Part model, mm, in its own coordinate system. Face numbers are marked on the shaded views. A direction names the side the tool comes from. Round coordinates to 2 decimals unless told otherwise and drop trailing zeros. Write each loop counter-clockwise with the first axis right and the second up, starting at its lowest first coordinate (ties: lowest second). Pieces come first, ordered by that corner, then holes. Notation, with made-up numbers: (30.25, 6) -> (48.25, 6) arc R11 ccw to (48.25, 19) -> close; hole circle Ø9 at (52, 54.5). An arc over 180 degrees is marked (long way). Use CSV: the item, a comma, the result in double quotes. Start each with the question number.
(1) Two-plate mould, pull along Z, no slides. Class the marked faces 1, 2 and 3: released by +Z, released by -Z, zero draft, split by the parting line, or undercut.
(2) Saw through at C-C (x = 6.5). Give the cut face in (y, z).
(3) Saw through at A-A (z = 0). Give the cut face in (x, y), plus the area to 3 significant figures.
(4) Probe line 1 (Z direction, x = 6.25, y = 0); line 2 (X direction, y = -4.5, z = -2); line 3 (Y direction, x = 11, z = 2.75). List the from-to ranges inside material, lowest first. Write a range as [from, to].
(5) Which spindle directions (+Z, -Z, +X, -X, +Y, -Y) get a long thin tool onto all of the face, cutting with end or side? Do the marked faces 4 and 5. Say none if no direction does.
(6) Saw through at D-D (y = -5). Give the cut face in (x, z).
(7) Drop flat-ended pins along their axis: pin 1 (2 mm diameter, centred on x = 1.5, y = -1, fed in from +Z); pin 2 (1 mm diameter, centred on x = 9.5, z = -3.5, fed in from +Y); pin 3 (4 mm diameter, centred on x = 1, z = -4.5, fed in from -Y). Give the stop position or say it passes through.
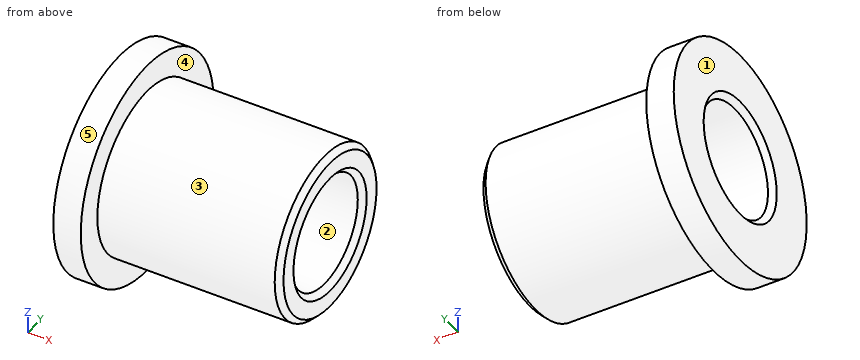
Autodesk Inventor part; units mm, degrees
ref_plane "YZ Plane" through (0, 0, 0) normal (1, 0, 0) x (0, 1, 0)
ref_plane "XZ Plane" through (0, 0, 0) normal (0, 1, 0) x (-1, 0, 0)
ref_plane "XY Plane" through (0, 0, 0) normal (0, 0, 1) x (1, 0, 0)
sketch "Sketch_1" plane through (0, 0, 0) normal (0, 0, 1) x (1, 0, 0)
  line L0 (11.5, 0) -> (0, 0)
  line L1 (0, 6) -> (0, 3.3)
  line L2 (0, 3.3) -> (0.3, 3)
  line L3 (0.3, 3) -> (11.2, 3)
  line L4 (11.2, 3) -> (11.5, 3.3)
  line L5 (11.5, 3.3) -> (11.5, 4.2)
  line L6 (11.5, 4.2) -> (11.2, 4.5)
  line L7 (11.2, 4.5) -> (1.5, 4.5)
  line L8 (1.5, 4.5) -> (1.5, 6)
  line L9 (1.5, 6) -> (0, 6)
revolve "Revolution1" add sketch "Sketch_1" angle 360 about axis through (11.5, 0, 0) along (1, 0, 0)
properties part number "TFZF6-10"
Answers:
1,face 1,"zero draft"
1,face 2,"undercut"
1,face 3,"split by the parting line"
2,outline,"circle Ø9 at (0, 0); hole circle Ø6 at (0, 0)"
3,outline,"(0, -6) -> (1.5, -6) -> (1.5, -4.5) -> (11.2, -4.5) -> (11.5, -4.2) -> (11.5, -3.3) -> (11.2, -3) -> (0.3, -3) -> (0, -3.3) -> close; (0, 3.3) -> (0.3, 3) -> (11.2, 3) -> (11.5, 3.3) -> (11.5, 4.2) -> (11.2, 4.5) -> (1.5, 4.5) -> (1.5, 6) -> (0, 6) -> close"
3,area,"38.7 mm²"
4,line 1,"z = [-4.5, -3], [3, 4.5]"
4,line 2,"x = [0, 1.5]"
4,line 3,"y = [-3.56, -1.2], [1.2, 3.56]"
5,face 4,"+X"
5,face 5,"+X, -X"
6,outline,"(0, -3.32) -> (1.5, -3.32) -> (1.5, 3.32) -> (0, 3.32) -> close"
7,pin 1,"stops at z = 6"
7,pin 2,"stops at y = 3.35"
7,pin 3,"stops at y = -5.45"
